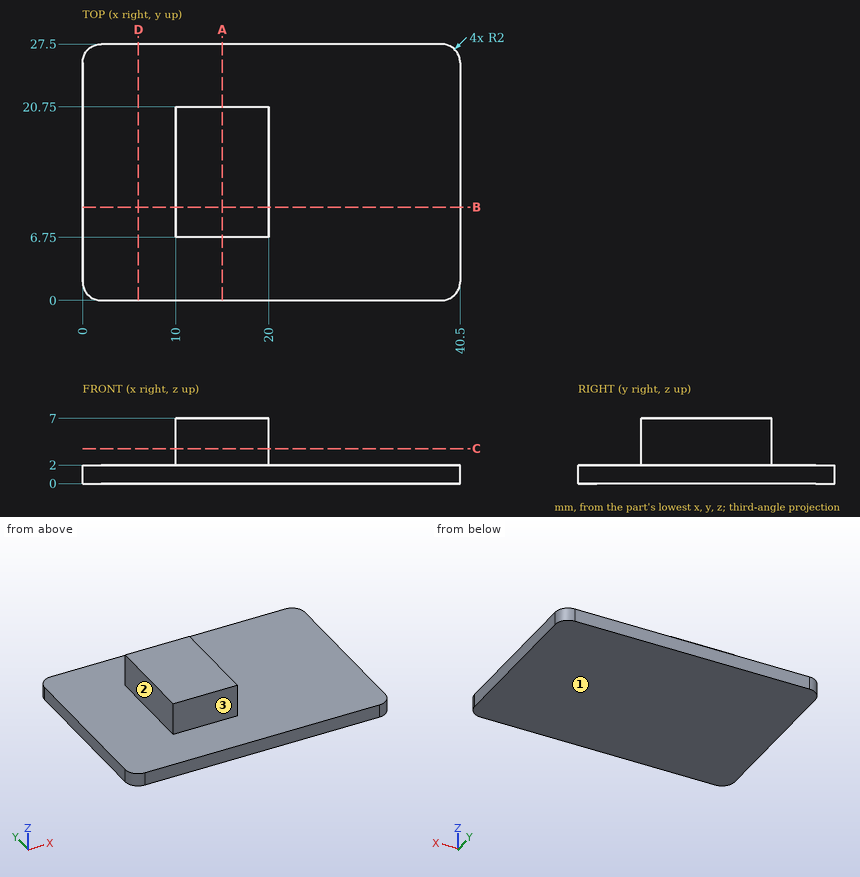
Part print with two shaded views. Sizes in mm from the minimum x, y, z corner. A direction names the side the tool comes from. Coordinates: 2 decimals unless noted, no trailing zeros. Order: outer loops, then holes, each group sorted by start corner. A loop starts at its lowest first (then second) coordinate and runs counter-clockwise, first axis right, second up. Notation, with made-up numbers: (15.25, 56) - (56.25, 56) arc R18 ccw to (56.25, 81) - close; hole circle Ø11 at (-10.5, -10). An arc over 180 degrees is marked (long way). Answer in a Markdown table with one row per item.
1. Slice it at D-D, the plane x = 6. List the corners of the cut face in (y, z).
Answer:
| item | result |
|---|---|
| outline | (0, 0) - (27.5, 0) - (27.5, 2) - (0, 2) - close |
2. Slice it at B-B, the plane y = 10. List the corners of the cut face in (x, z), then the cut area to 3 significant figures.
Answer:
| item | result |
|---|---|
| outline | (0, 0) - (40.5, 0) - (40.5, 2) - (20, 2) - (20, 7) - (10, 7) - (10, 2) - (0, 2) - close |
| area | 131 mm² |
3. Flat gauge pins, fed straight in: P1, Ø3, axis at x = 17, z = 5.5, coming from the +Y side; P2, Ø4, axis at y = 7.5, z = 5, coming from the -X side; P3, Ø4, axis at y = 20.5, z = 1, coming from the -X side; P4, Ø4, axis at x = 15.5, z = 4.5, coming from the -Y side. Where does each tip first touch, or does it go through?
Answer:
| item | result |
|---|---|
| P1 | y = 20.75 |
| P2 | x = 10 |
| P3 | x = 0 |
| P4 | y = 6.75 |
4. Drill centre lines: L1, parallel to Z at x = 27.5, y = 21; L2, parallel to X at y = 10.25, z = 6.25; L3, parallel to Y at x = 17.5, z = 5.75. Where is each one in solid material? Low to high. Write a range as from..to.
Answer:
| item | result |
|---|---|
| L1 | 0..2 |
| L2 | 10..20 |
| L3 | 6.75..20.75 |
5. Slice it at C-C, the plane z = 3.75. List the corners of the cut face in (x, y).
Answer:
| item | result |
|---|---|
| outline | (10, 6.75) - (20, 6.75) - (20, 20.75) - (10, 20.75) - close |
6. Slice it at A-A, the plane x = 15. List the corners of the cut face in (y, z), then the cut area to 3 significant figures.
Answer:
| item | result |
|---|---|
| outline | (0, 0) - (27.5, 0) - (27.5, 2) - (20.75, 2) - (20.75, 7) - (6.75, 7) - (6.75, 2) - (0, 2) - close |
| area | 125 mm² |
7. 3-axis set-ups, long thin cutter, end or side, ignore diameter. For the marked faces 1, 2 and 3: which of +Z, -Z, +X, -X, +Y, -Y reach the whole face in a straight line?
Answer:
| item | result |
|---|---|
| face 1 | -Z, +X, -X, +Y, -Y |
| face 2 | +Z, -X, +Y, -Y |
| face 3 | +Z, +X, -X, -Y |
